For this review, use the dimensioned drawing (mm, ordinates from the lowest corner) and the shaded views. A direction names the side the tool comes from. Round coordinates to 2 decimals unless told otherwise and drop trailing zeros. Loops run counter-clockwise (first coordinate to the right, second up) from the corner with the lowest first, then second, coordinate; pieces in that order, holes last. Notation, with made-up numbers: (30.25, 44) - (62.25, 44) arc R16 ccw to (62.25, 53) - close; hole circle Ø7 at (81, 31). An arc over 180 degrees is marked (long way). Answer as CSV lines item,"result". Start each with the question number.
(1) Consider section C-C (x = 117.5). Give the boundary of the cut face in (y, z), and give its area (3 significant figures).
(2) For the marked faces 4 and 5, list the 3-axis set-ups (+Z, -Z, +X, -X, +Y, -Y) from which the entire face can be reached by the end or side of a thin tool; tool diameter is ignored.
(3) Wall thickness on L1, parallel to X at y = 23.5, z = 3; L2, parallel to Z at x = 70, y = 93.5; L3, parallel to X at y = 136, z = 48.5: over which ranges is each line inside the solid? List them lowest first.
(4) Consider section B-B (y = 238.5). Give the boundary of the cut face in (x, z), and give its area (3 significant figures).
(5) Mouldability with a two-part tool opening along X and no side actions: class the marked faces 1, 2 and 3 as released by +X, released by -X, zero draft, split by the parting line, or undercut.
(6) For P1, Ø1, axis at x = 92, y = 147.5, coming from the -Z side, flat-tipped, find the tip position at first contact; note if it passes through.
(7) Consider section A-A (z = 17.5). Give the boundary of the cut face in (x, y), and give its area (3 significant figures).
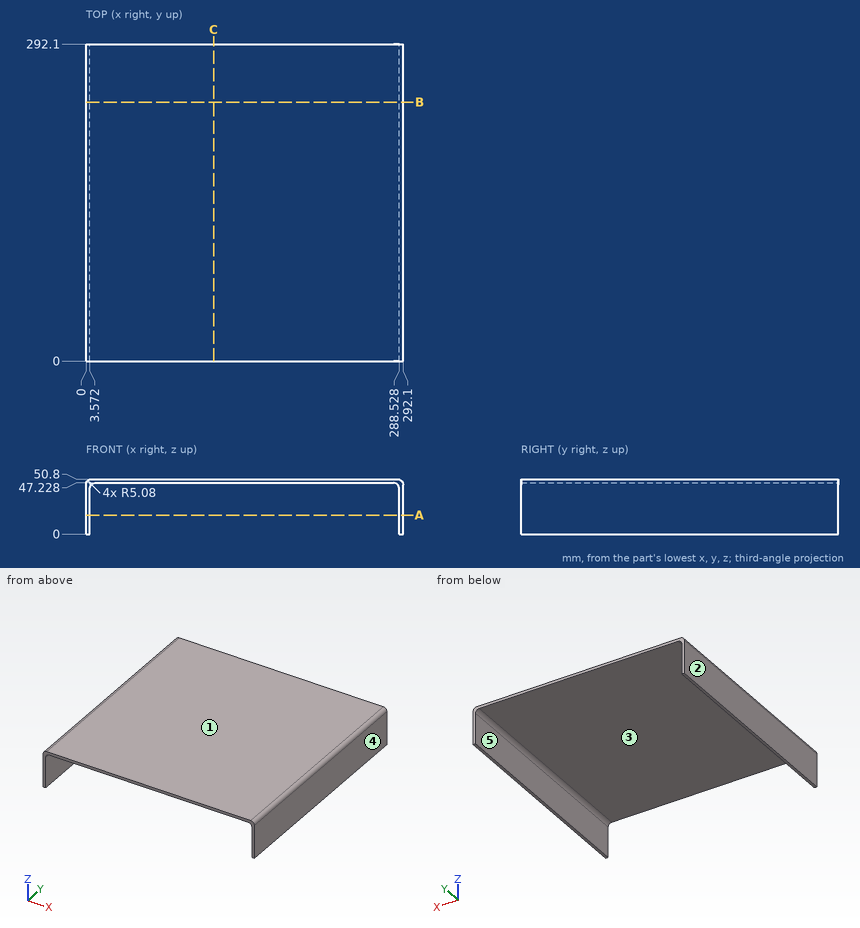
Determined:
1,outline,"(0, 47.23) - (292.1, 47.23) - (292.1, 50.8) - (0, 50.8) - close"
1,area,"1,040 mm^2"
2,face 4,"+Z, -Z, +X, +Y, -Y"
2,face 5,"-Z, +Y, -Y"
3,L1,"x = 0 to 3.57, 288.53 to 292.1"
3,L2,"z = 47.23 to 50.8"
3,L3,"x = 0.83 to 291.27"
4,outline,"(0, 0) - (3.57, 0) - (3.57, 42.15) arc R5.08 cw to (8.65, 47.23) - (283.45, 47.23) arc R5.08 cw to (288.53, 42.15) - (288.53, 0) - (292.1, 0) - (292.1, 45.72) arc R5.08 ccw to (287.02, 50.8) - (5.08, 50.8) arc R5.08 ccw to (0, 45.72) - close"
4,area,"1,380 mm^2"
5,face 1,"zero draft"
5,face 2,"released by -X"
5,face 3,"undercut"
6,P1,"stops at z = 47.23"
7,outline,"(0, 0) - (3.57, 0) - (3.57, 292.1) - (0, 292.1) - close; (288.53, 0) - (292.1, 0) - (292.1, 292.1) - (288.53, 292.1) - close"
7,area,"2,090 mm^2"
